Input: part model. Units: mm. Frame: model coordinates. Face numbers are marked on the shaded views. Round coordinates to 2 decimals unless told otherwise and drop trailing zeros. Order: outer loops, then holes, each group sorted by start corner. A loop starts at its lowest first (then second) coordinate and runs counter-clockwise, first axis right, second up. Notation, with made-up numbers: (36, 4) -> (85, 4) arc R20 ccw to (85, 28) -> close; hole circle Ø1 at (30.5, 19.25). An arc over 180 degrees is marked (long way). Use a Markdown table: item, result.
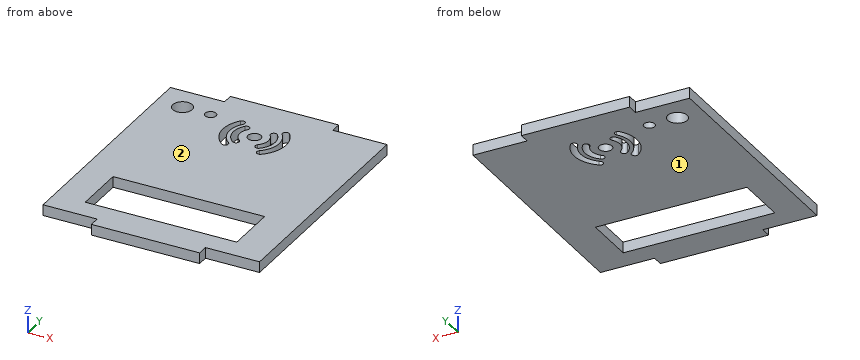
from build123d import *

# Parameters (mm, degrees)
SKETCH1_R           = 4.5
SKETCH1_R_2         = 3
SKETCH1_R_3         = 2.5
SKETCH1_W           = 70
SKETCH1_H           = 24
BOSS_EXTRUDE1_DEPTH = 5


with BuildPart() as part:
    # Sketch1 → Boss-Extrude1 (new body)
    with BuildSketch(Plane.XY):
        Polygon((-24.143882276, 60), (25.856117724, 60), (25.856117724, 55), (50.856117724, 55), (50.856117724, -55), (25.856117724, -55), (25.856117724, -60), (-24.143882276, -60), (-24.143882276, -55), (-49.143882276, -55), (-49.143882276, 55), (-24.143882276, 55), align=None)
        with Locations((-37.143882276, 43)):
            Circle(SKETCH1_R, mode=Mode.SUBTRACT)
        with Locations((0.348837209, 35)):
            Circle(SKETCH1_R_2, mode=Mode.SUBTRACT)
        with Locations((-24.143882276, 43)):
            Circle(SKETCH1_R_3, mode=Mode.SUBTRACT)
        with Locations((0, -33)):
            Rectangle(SKETCH1_W, SKETCH1_H, mode=Mode.SUBTRACT)
        with BuildLine():
            ThreePointArc((6.483996619, 27.71689355), (9.83698399, 34.188278863), (7.631943659, 41.13515941))
            ThreePointArc((7.631943659, 41.13515941), (5.486209752, 41.318729247), (5.302639914, 39.17299534))
            ThreePointArc((5.302639914, 39.17299534), (6.802457997, 34.447885818), (4.521832549, 30.046197295))
            ThreePointArc((4.521832549, 30.046197295), (4.338262711, 27.900463388), (6.483996619, 27.71689355))
        make_face(mode=Mode.SUBTRACT)
        with BuildLine():
            ThreePointArc((-7.289461523, 40.990419638), (-9.288121969, 33.834773518), (-5.641582428, 27.361701268))
            ThreePointArc((-5.641582428, 27.361701268), (-3.535600715, 27.61634027), (-3.790239716, 29.722321983))
            ThreePointArc((-3.790239716, 29.722321983), (-6.309814067, 34.194887447), (-4.928840807, 39.139076925))
            ThreePointArc((-4.928840807, 39.139076925), (-5.183479809, 41.245058639), (-7.289461523, 40.990419638))
        make_face(mode=Mode.SUBTRACT)
        with BuildLine():
            ThreePointArc((-10.994860864, 44.031639609), (-14.058702235, 33.365127781), (-8.6828024, 23.656301927))
            ThreePointArc((-8.6828024, 23.656301927), (-6.575008846, 23.895480389), (-6.814187308, 26.003273942))
            ThreePointArc((-6.814187308, 26.003273942), (-11.077832005, 33.703377206), (-8.647888849, 42.163024517))
            ThreePointArc((-8.647888849, 42.163024517), (-8.887067311, 44.270818071), (-10.994860864, 44.031639609))
        make_face(mode=Mode.SUBTRACT)
        with BuildLine():
            ThreePointArc((9.373364684, 23.607418094), (14.785913704, 33.325532654), (11.741419115, 44.024527475))
            ThreePointArc((11.741419115, 44.024527475), (9.586661553, 44.274444498), (9.33674453, 42.119686935))
            ThreePointArc((9.33674453, 42.119686935), (11.738626336, 33.678968697), (7.468524145, 26.01209268))
            ThreePointArc((7.468524145, 26.01209268), (7.218607122, 23.857335117), (9.373364684, 23.607418094))
        make_face(mode=Mode.SUBTRACT)
    extrude(amount=BOSS_EXTRUDE1_DEPTH)


solid = part.part
1) Cut plane D-D on z = 3.3. State how many separate pieces and enclosed holes the cut face has, and give its area (3 significant figures).
Answer key:
| item | result |
|---|---|
| separate pieces | 1 |
| enclosed holes | 8 |
| area | 9,480 mm^2 |
2) Cut plane B-B on x = -19.5. Return loops of the section in (y, z).
Answer key:
| item | result |
|---|---|
| outline | (-60, 0) -> (-45, 0) -> (-45, 5) -> (-60, 5) -> close; (-21, 0) -> (60, 0) -> (60, 5) -> (-21, 5) -> close |
3) Draft query along Z for the marked faces 1 and 2. Return one class per face: released by +Z, released by -Z, zero draft, split by the parting line, or undercut.
Answer key:
| item | result |
|---|---|
| face 1 | released by -Z |
| face 2 | released by +Z |
4) Cut plane A-A on y = 35. Return loops of the section in (x, z).
Answer key:
| item | result |
|---|---|
| outline | (-49.14, 0) -> (-14.15, 0) -> (-14.15, 5) -> (-49.14, 5) -> close; (-11.15, 0) -> (-9.36, 0) -> (-9.36, 5) -> (-11.15, 5) -> close; (-6.36, 0) -> (-2.65, 0) -> (-2.65, 5) -> (-6.36, 5) -> close; (3.35, 0) -> (6.83, 0) -> (6.83, 5) -> (3.35, 5) -> close; (9.87, 0) -> (11.81, 0) -> (11.81, 5) -> (9.87, 5) -> close; (14.88, 0) -> (50.86, 0) -> (50.86, 5) -> (14.88, 5) -> close |
5) Ray query, probe 1 along Y at (x, z) = (32, 2.2); probe 2 along Y at (x, z) = (-2, 3.95); probe 3 along X at (y, z) = (45, 2.5). Return the intervals inside material, ascending.
Answer key:
| item | result |
|---|---|
| probe 1 | y = -55 to -45, -21 to 55 |
| probe 2 | y = -60 to -45, -21 to 33.13, 36.87 to 60 |
| probe 3 | x = -49.14 to -41.18, -33.11 to -25.64, -22.64 to 50.86 |
6) Contact query for flat-ended pins moving along their axis: P1, Ø1.5, axis at x = -41, z = 2.5, coming from the +Y side; P2, Ø1.5, axis at x = -37, z = 3, coming from the -Y side; P3, Ø1.5, axis at y = 57.5, z = 1.5, coming from the -X side. Output: stop coordinate, or through.
Answer key:
| item | result |
|---|---|
| P1 | stops at y = 55 |
| P2 | stops at y = -55 |
| P3 | stops at x = -24.14 |
7) Cut plane C-C on x = -30. Return loops of the section in (y, z), and give its area (3 significant figures).
Answer key:
| item | result |
|---|---|
| outline | (-55, 0) -> (-45, 0) -> (-45, 5) -> (-55, 5) -> close; (-21, 0) -> (55, 0) -> (55, 5) -> (-21, 5) -> close |
| area | 430 mm^2 |
